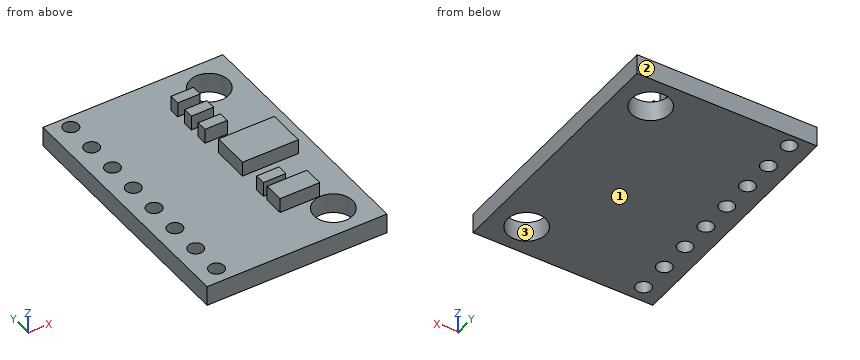
from build123d import *

# Parameters (mm, degrees)
SKETCH1_W           = 14.5
SKETCH1_H           = 20.5
BOSS_EXTRUDE1_DEPTH = 1.62
SKETCH2_R           = 1.55
CUT_EXTRUDE1_DEPTH  = 1.62
SKETCH3_W           = 1.8
SKETCH3_H           = 0.85
SKETCH3_W_2         = 4.5
SKETCH3_H_2         = 3
SKETCH3_W_3         = 3.2
SKETCH3_H_3         = 1.6
BOSS_EXTRUDE2_DEPTH = 1.2
SKETCH4_R           = 0.607226872
CUT_EXTRUDE2_DEPTH  = 13.658965203


with BuildPart() as part:
    # Sketch1 → Boss-Extrude1 (new body)
    with BuildSketch(Plane.XY):
        Rectangle(SKETCH1_W, SKETCH1_H)
    extrude(amount=BOSS_EXTRUDE1_DEPTH)

    # Sketch2 → Cut-Extrude1 (cut)
    with BuildSketch(Plane.XY.offset(1.62)):
        with Locations((4.54, 7.75)):
            Circle(SKETCH2_R)
        with Locations((4.54, -7.75)):
            Circle(SKETCH2_R)
    extrude(amount=-CUT_EXTRUDE1_DEPTH, mode=Mode.SUBTRACT)

    # Sketch3 → Boss-Extrude2 (add)
    with BuildSketch(Plane.XY.offset(1.62)):
        with Locations((1.94, 6.69017984)):
            Rectangle(SKETCH3_W, SKETCH3_H)
        with Locations((1.94, 4.99017984)):
            Rectangle(SKETCH3_W, SKETCH3_H)
        with Locations((1.94, 3.29017984)):
            Rectangle(SKETCH3_W, SKETCH3_H)
        with Locations((3.5, 0)):
            Rectangle(SKETCH3_W_2, SKETCH3_H_2)
        with Locations((2.15, -3.68482016)):
            Rectangle(SKETCH3_W, SKETCH3_H)
        with Locations((2.85, -5.38482016)):
            Rectangle(SKETCH3_W_3, SKETCH3_H_3)
    extrude(amount=BOSS_EXTRUDE2_DEPTH)

    # Sketch4 → Cut-Extrude2 (cut, through all)
    with BuildSketch(Plane.XY.offset(1.62)):
        with Locations((-5.65, 9.25)):
            Circle(SKETCH4_R)
        with Locations((-5.65, 6.65)):
            Circle(SKETCH4_R)
        with Locations((-5.65, 4.05)):
            Circle(SKETCH4_R)
        with Locations((-5.65, 1.45)):
            Circle(SKETCH4_R)
        with Locations((-5.65, -1.15)):
            Circle(SKETCH4_R)
        with Locations((-5.65, -3.75)):
            Circle(SKETCH4_R)
        with Locations((-5.65, -6.35)):
            Circle(SKETCH4_R)
        with Locations((-5.65, -8.95)):
            Circle(SKETCH4_R)
        with Locations((-5.65, -11.55)):
            Circle(SKETCH4_R)
        with Locations((-5.65, -14.15)):
            Circle(SKETCH4_R)
    extrude(amount=-CUT_EXTRUDE2_DEPTH, mode=Mode.SUBTRACT)


solid = part.part
Input: part model. Units: mm. Frame: model coordinates. Face numbers are marked on the shaded views. Round coordinates to 2 decimals unless told otherwise and drop trailing zeros. Order: outer loops, then holes, each group sorted by start corner. A loop starts at its lowest first (then second) coordinate and runs counter-clockwise, first axis right, second up. Notation, with made-up numbers: (4.25, -9.5) - (60.25, -9.5) arc R10 ccw to (60.25, -5.5) - close; hole circle Ø3 at (68, -3.75). An arc over 180 degrees is marked (long way). Use a Markdown table: item, result.
1. Section B-B on z = 0.5. State how many separate pieces and enclosed holes the cut face has, then the cut area to 3 significant figures.
Evaluation:
| item | result |
|---|---|
| separate pieces | 1 |
| enclosed holes | 10 |
| area | 273 mm^2 |
2. Material intervals for probe 1 along Y at (x, z) = (1.75, 1.75); probe 2 along Y at (x, z) = (3, 1.95); probe 3 along Y at (x, z) = (4.54, 0.9), sorted ascending.
Evaluation:
| item | result |
|---|---|
| probe 1 | -6.18 to -4.58, -4.11 to -3.26, -1.5 to 1.5, 2.87 to 3.72, 4.57 to 5.42, 6.27 to 7.12 |
| probe 2 | -6.18 to -4.58, -4.11 to -3.26, -1.5 to 1.5 |
| probe 3 | -10.25 to -9.3, -6.2 to 6.2, 9.3 to 10.25 |
3. Section C-C on x = 3.5. Return the cut outline in (y, z).
Evaluation:
| item | result |
|---|---|
| outline | (-10.25, 0) - (-8.9, 0) - (-8.9, 1.62) - (-10.25, 1.62) - close; (-6.6, 0) - (6.6, 0) - (6.6, 1.62) - (1.5, 1.62) - (1.5, 2.82) - (-1.5, 2.82) - (-1.5, 1.62) - (-4.58, 1.62) - (-4.58, 2.82) - (-6.18, 2.82) - (-6.18, 1.62) - (-6.6, 1.62) - close; (8.9, 0) - (10.25, 0) - (10.25, 1.62) - (8.9, 1.62) - close |
4. Section A-A on y = 7.75. Return the cut outline in (x, z).
Evaluation:
| item | result |
|---|---|
| outline | (-7.25, 0) - (2.99, 0) - (2.99, 1.62) - (-7.25, 1.62) - close; (6.09, 0) - (7.25, 0) - (7.25, 1.62) - (6.09, 1.62) - close |
5. Section D-D on z = 2.3. Return the cut outline in (x, y).
Evaluation:
| item | result |
|---|---|
| outline | (1.04, 2.87) - (2.84, 2.87) - (2.84, 3.72) - (1.04, 3.72) - close; (1.04, 4.57) - (2.84, 4.57) - (2.84, 5.42) - (1.04, 5.42) - close; (1.04, 6.27) - (2.84, 6.27) - (2.84, 7.12) - (1.04, 7.12) - close; (1.25, -6.18) - (4.45, -6.18) - (4.45, -4.58) - (1.25, -4.58) - close; (1.25, -4.11) - (3.05, -4.11) - (3.05, -3.26) - (1.25, -3.26) - close; (1.25, -1.5) - (5.75, -1.5) - (5.75, 1.5) - (1.25, 1.5) - close |
6. Mould query, pull axis Y, two halves, no side actions, for the marked faces 1, 2 and 3. Classes: +Y half, -Y half, draft (parallel to the pull), parting line (faces both ways), or undercut.
Evaluation:
| item | result |
|---|---|
| face 1 | draft |
| face 2 | +Y half |
| face 3 | undercut |
7. First-contact query: pin 1 (1.4 mm diameter, centred on x = -5.65, y = -1.15, fed in from +Z); pin 2 (4 mm diameter, centred on x = 4.54, y = 7.75, fed in from +Z); pin 3 (0.7 mm diameter, centred on y = -4, z = 2, fed in from -X); pin 4 (1 mm diameter, centred on x = 3.5, z = 2.5, fed in from +Y). Flat tips, straight axial feed; report the tip coordinate or a pass-through.
Evaluation:
| item | result |
|---|---|
| pin 1 | z = 1.62 |
| pin 2 | z = 2.82 |
| pin 3 | x = 1.25 |
| pin 4 | y = 1.5 |
